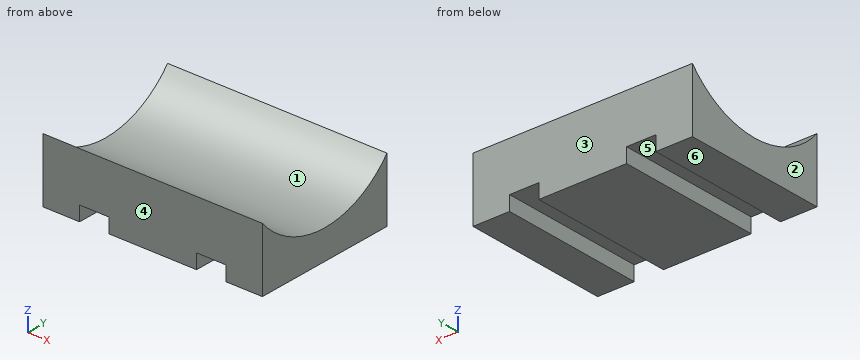
Autodesk Fusion 360 part; units mm, degrees
sketch "Sketch1" plane through (0, 0, 0) normal (0, 0, 1) x (1, 0, 0)
sketch "Sketch2" plane through (0, 0, 0) normal (0, 0, 1) x (1, 0, 0)
  line L0 (0, 0) -> (30, 0)
  line L1 (30, 0) -> (30, 20)
  line L2 (30, 20) -> (0, 20)
  line L3 (0, 20) -> (0, 0)
  dimension "d1" = 30
  dimension "d2" = 20
extrude "Extrude1" add sketch "Sketch2" along normal blind 15
sketch "Sketch3" plane through (30, 0, 0) normal (1, 0, 0) x (0, 1, 0)
  line L0 (0, 0) -> (20, 0)
  line L1 (20, 0) -> (20, 15)
  line L2 (20, 15) -> (0, 15)
  line L3 (0, 15) -> (0, 0)
  circle A0 centre (10, 17) radius 13
  dimension "d5" = 26
  dimension "d6" = 17
  dimension "d7" = 10
extrude "Extrude2" cut sketch "Sketch3" against normal blind 60 contours L1 L2 L3 A0 | L1 L2 L3 A0
sketch "Sketch4" plane through (0, 0, 0) normal (0, -1, 0) x (1, 0, 0)
  line L0 (30, 8.6934) -> (0, 8.6934)
  line L1 (0, 8.6934) -> (0, 0)
  line L2 (0, 0) -> (30, 0)
  line L3 (30, 0) -> (30, 8.6934)
  line L4 (5, 0) -> (9, 0)
  line L5 (9, 0) -> (9, 2)
  line L6 (9, 2) -> (5, 2)
  line L7 (5, 2) -> (5, 0)
  line L8 (21, 0) -> (25, 0)
  line L9 (25, 0) -> (25, 2)
  line L10 (25, 2) -> (21, 2)
  line L11 (21, 2) -> (21, 0)
  dimension "d10" = 4
  dimension "d11" = 2
  dimension "d12" = 4
  dimension "d13" = 2
  dimension "d14" = 5
  dimension "d15" = 5
extrude "Extrude3" cut sketch "Sketch4" against normal blind 50 contours L2 L8 L9 L10 L11 | L2 L4 L5 L6 L7
Here's how the part is built. I have some questions about the finished solid (model axes, mm). Face numbers are marked on the shaded views. A direction names the side the tool comes from. Coordinates: 2 decimals unless noted, no trailing zeros. Order: outer loops, then holes, each group sorted by start corner. A loop starts at its lowest first (then second) coordinate and runs counter-clockwise, first axis right, second up.
Item 1: For the marked faces 5 and 6, which set-ups out of +Z, -Z, +X, -X, +Y, -Y let a thin tool reach every point of the face, with its end or its side?
Result sheet:
face 5: -Z, +Y, -Y
face 6: -Z, +X, -X, +Y, -Y
Item 2: If we section it at C-C on z = 1: List the corners of the cut face in (x, y) for me.
Result sheet:
outline: (0, 0) - (5, 0) - (5, 20) - (0, 20) - close; (9, 0) - (21, 0) - (21, 20) - (9, 20) - close; (25, 0) - (30, 0) - (30, 20) - (25, 20) - close
Item 3: If we section it at A-A on z = 5: List the corners of the cut face in (x, y) for me.
Result sheet:
outline: (0, 0) - (30, 0) - (30, 5) - (0, 5) - close; (0, 15) - (30, 15) - (30, 20) - (0, 20) - close
Item 4: If we section it at B-B on y = 10: List the corners of the cut face in (x, z) for me, plus the area to 3 significant figures.
Result sheet:
outline: (0, 0) - (5, 0) - (5, 2) - (9, 2) - (9, 0) - (21, 0) - (21, 2) - (25, 2) - (25, 0) - (30, 0) - (30, 4) - (0, 4) - close
area: 104 mm2
Item 5: If we mould it in two halves opening along Y, with no side actions, what happens to the marked faces 1, 2, 3 and 4? For each: +Y half, -Y half, draft (parallel to the pull), parting line (faces both ways), or undercut.
Result sheet:
face 1: undercut
face 2: draft
face 3: +Y half
face 4: -Y half
Item 6: For P1, Ø8, axis at x = 19, y = 7, coming from the +Z side; P2, Ø3, axis at y = 6.5, z = 7, coming from the -X side; P3, Ø3, axis at x = 21, y = 17, coming from the +Z side; P4, Ø1.2, axis at x = 23, y = 9.5, coming from the -Z side, each with a flat end and sliding along its axis, tell me the tip position at first contact or that it passes through.
Result sheet:
P1: stops at z = 6.05
P2: passes through
P3: stops at z = 7.16
P4: stops at z = 2
Item 7: If we section it at D-D on x = 7.75: List the corners of the cut face in (y, z) for me, plus the area to 3 significant figures.
Result sheet:
outline: (0, 2) - (20, 2) - (20, 8.69) arc R13 cw to (0, 8.69) - close
area: 68.6 mm2
Item 8: I need wall thicknesses on line 1 (X direction, y = 18, z = 0.75); line 2 (Y direction, x = 5.25, z = 5); line 3 (Y direction, x = 27, z = 5.75). Which ranges of each line are inside material? Lowest first, please.
Result sheet:
line 1: x = 0 to 5, 9 to 21, 25 to 30
line 2: y = 0 to 5, 15 to 20
line 3: y = 0 to 3.49, 16.51 to 20
